Check sheet for the modelled part. Datum: model origin and axes. Units: mm. A direction names the side the tool comes from. Coordinates: 2 decimals unless noted, no trailing zeros. Write each loop counter-clockwise with the first axis right and the second up, starting at its lowest first coordinate (ties: lowest second). Pieces come first, ordered by that corner, then holes. Notation, with made-up numbers: (87, 65) -> (93, 65) arc R17 ccw to (93, 69) -> close; hole circle Ø7 at (20, 56). An arc over 180 degrees is marked (long way). Put each result on its own line as item: value.
```python
from build123d import *

# Parameters (mm, degrees)
SKETCH_R          = 1.6
PAD_DEPTH         = 12.5
SKETCH001_W       = 9.5
SKETCH001_H       = 14
POCKET_DEPTH      = 17.501
POCKET_DEPTH_BACK = -17.501
SKETCH011_R       = 1.5
POCKET001_DEPTH   = 1
SKETCH012_W       = 0.5
SKETCH012_H       = 1
POCKET002_DEPTH   = 8
SKETCH013_W       = 3
SKETCH013_H       = 0.5
POCKET003_DEPTH   = 17
SKETCH014_W       = 3
SKETCH014_H       = 0.5
POCKET004_DEPTH   = 15


with BuildPart() as part:
    # Sketch → Pad (new body, symmetric)
    with BuildSketch(Plane.YZ):
        Polygon((-17.5, 0), (-17.5, 6.590108), (-14.5, 11.786261), (-3.6, 20), (7, 20), (17.5, 6.560613), (17.5, 0), align=None)
        with Locations((0, 14)):
            Circle(SKETCH_R, mode=Mode.SUBTRACT)
    extrude(amount=PAD_DEPTH, both=True)

    # Sketch001 → Pocket (cut, two sides)
    with BuildSketch(Plane.XZ) as pocket_sk:
        with Locations((0, 14)):
            Rectangle(SKETCH001_W, SKETCH001_H)
    extrude(amount=-POCKET_DEPTH, mode=Mode.SUBTRACT)
    extrude(pocket_sk.sketch, amount=-POCKET_DEPTH_BACK, mode=Mode.SUBTRACT)

    # Sketch002 → Groove (revolve, cut)
    with BuildSketch(Plane.XY.offset(14)):
        Polygon((-5, 0), (12.5, 0), (12.5, 3.1), (8, 3.1), (8, 1.6), (5, 1.6), (5, 10), (-5, 10), align=None)
    revolve(axis=Axis((-5, 0, 14), (1, 0, 0)), mode=Mode.SUBTRACT)

    # Sketch004 → SubtractiveLoft section 0
    with BuildSketch(Plane.YZ.offset(-10)):
        Polygon((-1.549897, 16.6845), (-3.099794, 14), (-1.549897, 11.3155), (1.549897, 11.3155), (3.099794, 14), (1.549897, 16.6845), align=None)
    # Sketch003 → SubtractiveLoft section 1
    with BuildSketch(Plane.YZ.offset(-12.5)):
        Polygon((-3.66271, 14), (-1.831355, 10.828), (1.831355, 10.828), (3.66271, 14), (1.831355, 17.172), (-1.831355, 17.172), align=None)
    loft(mode=Mode.SUBTRACT)

    # Sketch006 → SubtractiveLoft001 section 0
    with BuildSketch(Plane.XY.offset(5)):
        Polygon((-1.550185, -9.815), (-3.100371, -12.5), (-1.550185, -15.185), (1.550185, -15.185), (3.100371, -12.5), (1.550185, -9.815), align=None)
    # Sketch005 → SubtractiveLoft001 section 1
    with BuildSketch(Plane.XY.offset(7)):
        Polygon((-1.682976, -9.585), (-3.365952, -12.5), (-1.682976, -15.415), (1.682976, -15.415), (3.365952, -12.5), (1.682976, -9.585), align=None)
    loft(mode=Mode.SUBTRACT)

    # Sketch007 → Groove001 (revolve, cut)
    with BuildSketch(Plane.XZ.offset(12.5)):
        Polygon((0, 7), (-1.65, 7), (-1.65, 1), (-2.074475, 0), (0, 0), align=None)
    revolve(axis=Axis((0, -12.5, 0), (0, 0, 1)), mode=Mode.SUBTRACT)

    # Sketch008 → SubtractiveLoft002 section 0
    with BuildSketch(Plane.XY.offset(7)):
        Polygon((-1.682976, 16.415), (-3.365952, 13.5), (-1.682976, 10.585), (1.682976, 10.585), (3.365952, 13.5), (1.682976, 16.415), align=None)
    # Sketch009 → SubtractiveLoft002 section 1
    with BuildSketch(Plane.XY.offset(5)):
        Polygon((-1.550185, 16.185), (-3.100371, 13.5), (-1.550185, 10.815), (1.550185, 10.815), (3.100371, 13.5), (1.550185, 16.185), align=None)
    loft(mode=Mode.SUBTRACT)

    # Sketch010 → Groove002 (revolve, cut)
    with BuildSketch(Plane.XZ.offset(-13.5)):
        Polygon((0, 7), (-1.65, 7), (-1.65, 1), (-2.074475, 0), (0, 0), align=None)
    revolve(axis=Axis((0, 13.5, 0), (0, 0, 1)), mode=Mode.SUBTRACT)

    # Sketch011 (on Face6 of Groove002) → Pocket001 (cut)
    with BuildSketch(Plane.ZX.offset(17.5)):
        with Locations((3.5, 8.5)):
            Circle(SKETCH011_R)
    extrude(amount=-POCKET001_DEPTH, mode=Mode.SUBTRACT)

    # Sketch012 → Pocket002 (cut, symmetric)
    with BuildSketch(Plane.YZ):
        with Locations((-9.25, 1.5)):
            Rectangle(SKETCH012_W, SKETCH012_H)
        with Locations((7.75, 1.5)):
            Rectangle(SKETCH012_W, SKETCH012_H)
    extrude(amount=POCKET002_DEPTH, both=True, mode=Mode.SUBTRACT)

    # Sketch013 → Pocket003 (cut)
    with BuildSketch(Plane.XY.offset(1)):
        with Locations((-8.5, 4.75)):
            Rectangle(SKETCH013_W, SKETCH013_H)
        with Locations((9.5, 4.75)):
            Rectangle(SKETCH013_W, SKETCH013_H)
        with Locations((9.5, -4.25)):
            Rectangle(SKETCH013_W, SKETCH013_H)
        with Locations((-8.5, -4.25)):
            Rectangle(SKETCH013_W, SKETCH013_H)
    extrude(amount=POCKET003_DEPTH, mode=Mode.SUBTRACT)

    # Sketch014 → Pocket004 (cut)
    with BuildSketch(Plane.XY.offset(1)):
        with Locations((-8.5, 6.75)):
            Rectangle(SKETCH014_W, SKETCH014_H)
        with Locations((9.5, 6.75)):
            Rectangle(SKETCH014_W, SKETCH014_H)
        with Locations((9.5, -6.25)):
            Rectangle(SKETCH014_W, SKETCH014_H)
        with Locations((-8.5, -6.25)):
            Rectangle(SKETCH014_W, SKETCH014_H)
    extrude(amount=POCKET004_DEPTH, mode=Mode.SUBTRACT)


solid = part.part
```
Q1. Mould release check, pull along Z, two halves, no side actions. Record for faces 5 (the flat face through (2, 13, 5)), 6 (the cylindrical face through (0.4, -10.9, 3)), 7 (the flat face through (-0.1, -9, 1.5)): released by +Z, released by -Z, zero draft, split by the parting line, or undercut.
Recorded:
face 5: released by +Z
face 6: zero draft
face 7: undercut
Q2. Depth check by flat-ended pin: P1, Ø1.6, axis at x = 1, y = 12.5, coming from the +Z side; P2, Ø0.9, axis at x = 9, z = 10, coming from the -Y side; P3, Ø8, axis at x = -8.5, z = 14, coming from the -Y side. Enter the tip coordinate at first touch or a pass-through.
Recorded:
P1: stops at z = 5
P2: stops at y = -15.79
P3: stops at y = -15.53
Q3. Tool access check on faces 1 (the flat face through (-9, 2, 20)), 2 (the flat face through (-4.75, 12, 10)), 3 (the flat face through (-9, 4.5, 9)), 4 (the flat face through (2, -13, 5)). Record the directions out of +Z, -Z, +X, -X, +Y, -Y that give a thin tool (end or side, any length) a straight path to the whole face; none if there is none.
Recorded:
face 1: +Z, +X, -X, +Y, -Y
face 2: +Z, +Y, -Y
face 3: none
face 4: +Z
Q4. Cross-section at A-A (x = 8.5). Record the cut outline in (y, z), plus the area to 3 significant figures.
Recorded:
outline: (-17.5, 0) -> (17.5, 0) -> (17.5, 2) -> (16.5, 2) -> (16.5, 5) -> (17.5, 5) -> (17.5, 6.56) -> (7, 20) -> (-3.6, 20) -> (-14.5, 11.79) -> (-17.5, 6.59) -> close; hole (-6.5, 1) -> (-6, 1) -> (-6, 16) -> (-6.5, 16) -> close; hole (-4.5, 1) -> (-4, 1) -> (-4, 18) -> (-4.5, 18) -> close; hole circle Ø6.2 at (0, 14); hole (4.5, 1) -> (5, 1) -> (5, 18) -> (4.5, 18) -> close; hole (6.5, 1) -> (7, 1) -> (7, 16) -> (6.5, 16) -> close
area: 487 mm2
Q5. Cross-section at B-B (z = 9.5). State how many separate pieces and enclosed holes the cut face has, plus the area to 3 significant figures.
Recorded:
separate pieces: 2
enclosed holes: 8
area: 460 mm2
Q6. Cross-section at D-D (x = -9.25). Record the cut outline in (y, z), plus the area to 3 significant figures.
Recorded:
outline: (-17.5, 0) -> (17.5, 0) -> (17.5, 6.56) -> (7, 20) -> (-3.6, 20) -> (-14.5, 11.79) -> (-17.5, 6.59) -> close; hole (-6.5, 1) -> (-6, 1) -> (-6, 16) -> (-6.5, 16) -> close; hole (-4.5, 1) -> (-4, 1) -> (-4, 18) -> (-4.5, 18) -> close; hole circle Ø3.2 at (0, 14); hole (4.5, 1) -> (5, 1) -> (5, 18) -> (4.5, 18) -> close; hole (6.5, 1) -> (7, 1) -> (7, 16) -> (6.5, 16) -> close
area: 512 mm2
Q7. Material ranges on line 1 along Z through (x, y) = (9.35, 0); line 2 along Y through (x, z) = (-8, 8.75); line 3 along X through (y, z) = (-12.5, 12.25), recorded low to high.
Recorded:
line 1: z = 0 to 10.9, 17.1 to 20
line 2: y = -16.25 to -6.5, -6 to -4.5, -4 to 4.5, 5 to 6.5, 7 to 15.79
line 3: x = -12.5 to -4.75, 4.75 to 12.5
